Input: part model. Units: mm. Frame: model coordinates. A direction names the side the tool comes from. Coordinates: 2 decimals unless noted, no trailing zeros. Loops run counter-clockwise (first coordinate to the right, second up) from the corner with the lowest first, then second, coordinate; pieces in that order, holes last. Notation, with made-up numbers: (10, -11.75) - (35, -11.75) arc R15 ccw to (35, 17.25) - close; hole circle Ø11 at (-18.75, 19.25). An arc over 180 degrees is marked (long way). Use a Markdown table: item, result. Add a question column.
1. Draft query along Z for faces 1 (the face through (103.975, 322.524, 861.407)), 2 (the face through (112.356, 250, 798)), 3 (the face through (104, 176, -418.381)). Return one class per face: released by +Z, released by -Z, zero draft, split by the parting line, or undercut.
2. Section query C-C on x = 16. Return the cut outline in (y, z).
3. Section query B-B on z = -41. Return the cut outline in (x, y), then the cut area to 3 significant figures.
4. Ray query, L1, parallel to Z at x = 101, y = 333; L2, parallel to X at y = 339, z = 1214; L3, parallel to Y at x = -40, z = 1568. Return the intervals inside material, ascending. Write a range as [from, to].
5. Section query A-A on y = 333. Return the cut outline in (x, z), then the cut area to 3 significant figures.
6. Access query for faces 4 (the face through (95.356, 413, 798)), 5 (the face through (104, 176, 1981.619)). Directions: +Z, -Z, +X, -X, +Y, -Y. A direction counts if a zero-diameter tool reaches every point of the face in a straight line with its end or side. Return the directions, or none.
7. Contact query for flat-ended pins moving along their axis: P1, Ø4, axis at y = 156.5, z = 1506, coming from the -X side; P2, Ø6, axis at x = -236.5, z = 797, coming from the +Y side. Output: stop coordinate, or through.
8. Section query D-D on y = 107.5. Return the cut outline in (x, z).
```python
from build123d import *

# Parameters (mm, degrees)
F0_W     = 400
F0_H     = 2400
F1_DEPTH = 17
F2_W     = 700
F2_H     = 2400
F3_DEPTH = 17
F4_R     = 80.472245
F5_DEPTH = 25


with BuildPart() as f1:
    # F0 (on Front) → F1 (new body)
    with BuildSketch(Plane.XZ):
        with Locations((-104.643844, 781.619109)):
            Rectangle(F0_W, F0_H)
    extrude(amount=F1_DEPTH)

    # F2 (on face) → F3 (join)
    with BuildSketch(Plane.YZ.offset(95.356156)):
        with Locations((333, 781.619109)):
            Rectangle(F2_W, F2_H)
    extrude(amount=F3_DEPTH)

    # F4 (on face) → F5 (cut)
    with BuildSketch(Plane.YZ.offset(112.356156)):
        with Locations((333, 781.619109)):
            Circle(F4_R)
    extrude(amount=-F5_DEPTH, mode=Mode.SUBTRACT)


solid = f1.part
```
Resolved:
| question | item | result |
|---|---|---|
| 1 | face 1 | undercut |
| 1 | face 2 | zero draft |
| 1 | face 3 | released by -Z |
| 2 | outline | (-17, -418.38) - (0, -418.38) - (0, 1981.62) - (-17, 1981.62) - close |
| 3 | outline | (-304.64, -17) - (112.36, -17) - (112.36, 683) - (95.36, 683) - (95.36, 0) - (-304.64, 0) - close |
| 3 | area | 18,700 mm² |
| 4 | L1 | [-418.38, 701.15], [862.09, 1981.62] |
| 4 | L2 | [95.36, 112.36] |
| 4 | L3 | [-17, 0] |
| 5 | outline | (95.36, -418.38) - (112.36, -418.38) - (112.36, 701.15) - (95.36, 701.15) - close; (95.36, 862.09) - (112.36, 862.09) - (112.36, 1981.62) - (95.36, 1981.62) - close |
| 5 | area | 38,100 mm² |
| 6 | face 4 | +Z, -Z, -X, +Y |
| 6 | face 5 | +Z, +X, -X, +Y, -Y |
| 7 | P1 | x = 95.36 |
| 7 | P2 | y = 0 |
| 8 | outline | (95.36, -418.38) - (112.36, -418.38) - (112.36, 1981.62) - (95.36, 1981.62) - close |
